Part model, mm, in its own coordinate system. A direction names the side the tool comes from. Give positions to 0.01 mm unless a question says otherwise; leave off trailing zeros. Order: outer loops, then holes, each group sorted by start corner. A loop starts at its lowest first (then second) coordinate and runs counter-clockwise, first axis right, second up. Notation, with made-up numbers: M -7,32.25 L 52,32.25 A13 ccw 52,44.25 Z; hole C 51.5,34 d2. An arc over 180 degrees is marked long. One line per question, with ' | ' between items.
```python
from build123d import *

# Parameters (mm, degrees)
F0_R         = 26.25
F1_DEPTH     = 55
F2_R         = 52.5
F2_R_2       = 26.25
F3_DEPTH     = 10
F6_D         = 30
F6_DEPTH     = 40
F6_TIP       = 9.0129092854
F7_D         = 40
F7_DEPTH     = 30
F7_TIP       = 12.0172123806
F8_T10_ANGLE = 180
F8_T12_ANGLE = 180
F10_D        = 8.8


# Not quite as in the source:
# - a fillet or chamfer that OpenCascade refuses, or shapes differently, is made with other operations: its cross-section is extruded or revolved along the edge and cut away or added


with BuildPart() as f1:
    # F0 (on Front) → F1 (new body)
    with BuildSketch(Plane.XZ):
        Circle(F0_R)
    extrude(amount=F1_DEPTH)

    # F2 (on face) → F3 (join)
    with BuildSketch(Plane.XZ.offset(55)):
        Circle(F2_R)
        Circle(F2_R_2, mode=Mode.SUBTRACT)
        Circle(F2_R_2)
    extrude(amount=F3_DEPTH)

    # F6
    with Locations(Plane.XZ.offset(65)):
        with Locations((0, 0)):
            Hole(F6_D / 2, depth=F6_DEPTH)
            with Locations((0, 0, -(F6_DEPTH + F6_TIP / 2))):  # 118° drill point
                Cone(0, F6_D / 2, F6_TIP, mode=Mode.SUBTRACT)

    # F7
    with Locations(Plane(origin=(0, 0, 0), x_dir=(-1, 0, 0), z_dir=(0, 1, 0))):
        with Locations((0, 0)):
            Hole(F7_D / 2, depth=F7_DEPTH)
            with Locations((0, 0, -(F7_DEPTH + F7_TIP / 2))):  # 118° drill point
                Cone(0, F7_D / 2, F7_TIP, mode=Mode.SUBTRACT)

    # F8: chamfer of 1 on 7 edges, made by hand

    # F8_s1 → F8_t2 (revolve, cut)
    with BuildSketch(Plane.XY):
        Polygon((52.5, -56), (51.5, -55), (52.5, -55), align=None)
    revolve(axis=Axis((0, -55, 0), (0, -1, 0)), mode=Mode.SUBTRACT)

    # F8_s3 → F8_t4 (revolve, cut)
    with BuildSketch(Plane.XY):
        Polygon((26.25, -1), (25.25, 0), (26.25, 0), align=None)
    revolve(axis=Axis((0, 0, 0), (0, -1, 0)), mode=Mode.SUBTRACT)

    # F8_s5 → F8_t6 (revolve, cut)
    with BuildSketch(Plane.XY):
        Polygon((52.5, -64), (51.5, -65), (52.5, -65), align=None)
    revolve(axis=Axis((0, -65, 0), (0, -1, 0)), mode=Mode.SUBTRACT)

    # F8_s7 → F8_t8 (revolve, cut)
    with BuildSketch(Plane.XY):
        Polygon((16, -65), (15, -64), (15, -65), align=None)
    revolve(axis=Axis((0, -65, 0), (0, -1, 0)), mode=Mode.SUBTRACT)

    # F8_s9 → F8_t10 (revolve, cut)
    with BuildSketch(Plane.XY):
        Polygon((-15, -33.5700758733), (-15.4849619251, -32.7129085726), (-15, -33.0043030951), align=None)
    revolve(axis=Axis((0, -33.0043030951, 0), (0, -1, 0)), revolution_arc=F8_T10_ANGLE, mode=Mode.SUBTRACT)

    # F8_s11 → F8_t12 (revolve, cut)
    with BuildSketch(Plane.XY):
        Polygon((15, -33.5700758733), (15.4849619251, -32.7129085726), (15, -33.0043030951), align=None)
    revolve(axis=Axis((0, -33.0043030951, 0), (0, -1, 0)), revolution_arc=F8_T12_ANGLE, mode=Mode.SUBTRACT)

    # F8_s13 → F8_t14 (revolve, cut)
    with BuildSketch(Plane.XY):
        Polygon((-21, 0), (-20, -1), (-20, 0), align=None)
    revolve(axis=Axis((0, 0, 0), (0, 1, 0)), mode=Mode.SUBTRACT)

    # F10 (through all)
    with Locations(Plane.XZ.offset(65)):
        with Locations((0, 44.5)):
            Hole(F10_D / 2)


solid = f1.part
```
1. Tool access for faces 4 (the cylindrical face through (50.076, -59.944, 15.77)), 5 (the cylindrical face through (-4.336, -15.703, -19.524)): list every direction of +Z, -Z, +X, -X, +Y, -Y with a clear straight run to the whole face (end or side of a thin tool).
Worked out:
face 4: +Y, -Y | face 5: +Y
2. Probe L1, parallel to Z at x = 0, y = -59.25; L2, parallel to Z at x = 0, y = -20.5; L3, parallel to Z at x = 0, y = -46. List the from-to ranges inside material, lowest first. Write a range as from..to.
Worked out:
L1: z = -52.5..-15, 15..40.1, 48.9..52.5 | L2: z = -26.25..-20, 20..26.25 | L3: z = -26.25..-15, 15..26.25
3. Mould opens along Z. For faces 1 (the flat face through (-12, -65, -11)), 2 (the cylindrical face through (25, -28, 8)), 3 (the cylindrical face through (0.954, -59.93, 40.205)) say: released by +Z, released by -Z, zero draft, split by the parting line, or undercut.
Worked out:
face 1: zero draft | face 2: split by the parting line | face 3: undercut
4. Drop flat-ended pins along their axis: pin 1 (3 mm diameter, centred on x = 1, y = -10, fed in from -Z); pin 2 (10 mm diameter, centred on x = -8.5, y = -35.5, fed in from -Z); pin 3 (3 mm diameter, centred on x = -6.5, y = -40, fed in from -Z). Give the stop position or say it passes through.
Worked out:
pin 1: stops at z = -26.25 | pin 2: stops at z = -26.02 | pin 3: stops at z = -25.77
5. Slice it at A-A on x = 0. Give the number of separate pieces and of enclosed holes in the cut face, then the cut area to 3 significant figures.
Worked out:
separate pieces: 3 | enclosed holes: 0 | area: 1,580 mm2
6. Slice it at D-D on y = -50.5. Give the cut face in (x, z), then the cut area to 3 significant figures.
Worked out:
outline: C 0,0 d52.5; hole C 0,0 d30 | area: 1,460 mm2
7. Slice it at B-B on z = 0. Give the cut face in (x, y).
Worked out:
outline: M -52.5,-64 L -51.5,-65 L -16,-65 L -15,-64 L -15,-33.57 L -15.48,-32.71 L -20,-30 L -20,-1 L -21,0 L -25.25,0 L -26.25,-1 L -26.25,-55 L -51.5,-55 L -52.5,-56 Z; M 15,-64 L 16,-65 L 51.5,-65 L 52.5,-64 L 52.5,-56 L 51.5,-55 L 26.25,-55 L 26.25,-1 L 25.25,0 L 21,0 L 20,-1 L 20,-30 L 15.48,-32.71 L 15,-33.57 Z
8. Slice it at C-C on y = -17. Give the cut face in (x, z).
Worked out:
outline: C 0,0 d52.5; hole C 0,0 d40
